```python
from build123d import *

# Parameters (mm, degrees)
BOSS_EXTRUDE1_DEPTH   = 135
RIB3_REACH            = 95.436
SKETCH4_WALL_W        = 207.229173432
SKETCH4_WALL_H        = 3
RIB4_START            = -3
RIB4_DEPTH            = 3
F_6_CLEARANCE_HOLE1_D = 3.7973
SKETCH6_R             = 2.3495
CUT_EXTRUDE1_DEPTH    = 7
SKETCH12_R            = 2.6162
CUT_EXTRUDE2_DEPTH    = 6.35


# Read off the part's stored shape, not the designer's step: Rib4
with BuildPart() as part:
    # Sketch1 → Boss-Extrude1 (new body)
    with BuildSketch(Plane.XY):
        with BuildLine():
            Line((0, 0), (0, 12))
            Line((0, 12), (-8, 12))
            Line((-8, 12), (-8, 6))
            ThreePointArc((-8, 6), (-8.878679656, 3.878679656), (-11, 3))
            Line((-11, 3), (-24, 3))
            Line((-24, 3), (-24, 0))
            Line((-24, 0), (0, 0))
        make_face()
    extrude(amount=BOSS_EXTRUDE1_DEPTH)

    # Sketch4 wall → Rib3 (add, up to next)
    with BuildSketch(Plane(origin=(-16, 7.5, 45.5), x_dir=(-0.871575537125, -0.490261239633, 0), z_dir=(-0.490261239633, 0.871575537125, 0)), mode=Mode.PRIVATE) as rib3_sk1:
        Rectangle(SKETCH4_WALL_W, SKETCH4_WALL_H)
    rib3_tool1 = extrude(rib3_sk1.sketch, amount=-RIB3_REACH, mode=Mode.PRIVATE) - part.part
    rib3 = rib3_tool1.solids().sort_by_distance((-16, 7.5, 45.5))[0]
    add(rib3)

    # Rib4 outline → Rib4 (add)
    with BuildSketch(Plane(origin=(0, 0, 0), x_dir=(-1, 0, 0), z_dir=(0, 0, -1)).offset(RIB4_START)):
        with BuildLine():
            Line((24, 3), (8, 12))
            Line((8, 12), (8, 6))
            ThreePointArc((8, 6), (8.878679656, 3.878679656), (11, 3))
            Line((11, 3), (24, 3))
        make_face()
    rib4 = extrude(amount=RIB4_DEPTH)

    # Mirror1: Rib3, Rib4 across plane
    add(rib3.mirror(Plane(origin=(0, 0, 67.5), x_dir=(1, 0, 0), z_dir=(0, 0, -1))))
    add(rib4.mirror(Plane(origin=(0, 0, 67.5), x_dir=(1, 0, 0), z_dir=(0, 0, -1))))

    # #6 Clearance Hole1 (through all)
    with Locations(Plane(origin=(0, 0, 0), x_dir=(-1, 0, 0), z_dir=(0, -1, 0))):
        with Locations((17.5, -22.5), (17.5, -112.5), (17.5, -67.5)):
            Hole(F_6_CLEARANCE_HOLE1_D / 2)

    # Sketch6 → Cut-Extrude1 (cut)
    with BuildSketch(Plane(origin=(0, 0, 0), x_dir=(0, 0, -1), z_dir=(1, 0, 0))):
        with Locations((-112.5, 6)):
            Circle(SKETCH6_R)
        with Locations((-67.5, 6)):
            Circle(SKETCH6_R)
        with Locations((-22.5, 6)):
            Circle(SKETCH6_R)
    extrude(amount=-CUT_EXTRUDE1_DEPTH, mode=Mode.SUBTRACT)

    # Sketch12 → Cut-Extrude2 (cut)
    with BuildSketch(Plane(origin=(0, 0, 0), x_dir=(0, 0, -1), z_dir=(1, 0, 0))):
        with Locations((-112.5, 6)):
            Circle(SKETCH12_R)
        with Locations((-67.5, 6)):
            Circle(SKETCH12_R)
        with Locations((-22.5, 6)):
            Circle(SKETCH12_R)
    extrude(amount=-CUT_EXTRUDE2_DEPTH, mode=Mode.SUBTRACT)


solid = part.part
```
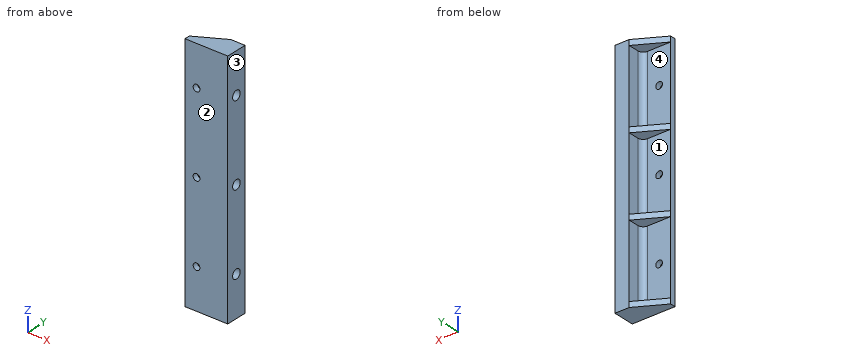
Source: CAD feature listing. Evaluate the final solid. Frame: model axes, mm. Face numbers are marked on the shaded views. A direction names the side the tool comes from. Round coordinates to 2 decimals unless told otherwise and drop trailing zeros. Loops run counter-clockwise (first coordinate to the right, second up) from the corner with the lowest first, then second, coordinate; pieces in that order, holes last.
(1) Section query B-B (z = 112.5). Output: boundary loops of the cut face in (x, y), and give its area (3 significant figures).
From the geometry:
outline: (-24, 0) - (-19.4, 0) - (-19.4, 3) - (-24, 3) - close; (-15.6, 0) - (0, 0) - (0, 3.38) - (-6.35, 3.38) - (-6.35, 3.65) - (-7, 3.65) - (-7, 8.35) - (-6.35, 8.35) - (-6.35, 8.62) - (0, 8.62) - (0, 12) - (-8, 12) - (-8, 6) arc R3 cw to (-11, 3) - (-15.6, 3) - close
area: 98.3 mm2
(2) Contact query for flat-ended pins moving along their axis: pin 1 Ø1.6 at (y, z) = (5, 68.5) entering from +X; pin 2 Ø10.5 at (x, z) = (-20, 109.5) entering from +Y; pin 3 Ø4 at (y, z) = (9.5, 91) entering from -X. Output: stop coordinate, or through.
From the geometry:
pin 1: stops at x = -7
pin 2: stops at y = 3
pin 3: stops at x = -16
(3) Access query for the marked faces 3 and 4. Directions: +Z, -Z, +X, -X, +Y, -Y. A direction counts if a zero-diameter tool reaches every point of the face in a straight line with its end or side. Return the directions, or none.
From the geometry:
face 3: +Z, -Z, +X, +Y, -Y
face 4: -X, +Y
(4) Pull-direction query (Z, two-part tool) for the marked faces 1 and 2; classes: +Z half, -Z half, draft (parallel to the pull), parting line (faces both ways), or undercut.
From the geometry:
face 1: undercut
face 2: draft
(5) Material intervals for probe 1 along Z at (x, y) = (-9, 7.5); probe 2 along Y at (x, z) = (-6.75, 112.5); probe 3 along Z at (x, y) = (-17.5, 1.8), sorted ascending.
From the geometry:
probe 1: z = 0 to 3, 44 to 47, 88 to 91, 132 to 135
probe 2: y = 0 to 3.65, 8.35 to 12
probe 3: z = 0 to 20.6, 24.4 to 65.6, 69.4 to 110.6, 114.4 to 135
(6) Section query A-A (x = -17.5). Output: boundary loops of the cut face in (y, z), and give its area (3 significant figures).
From the geometry:
outline: (0, 0) - (6.66, 0) - (6.66, 3) - (3, 3) - (3, 20.6) - (0, 20.6) - close; (0, 24.4) - (3, 24.4) - (3, 44) - (6.66, 44) - (6.66, 47) - (3, 47) - (3, 65.6) - (0, 65.6) - close; (0, 69.4) - (3, 69.4) - (3, 88) - (6.66, 88) - (6.66, 91) - (3, 91) - (3, 110.6) - (0, 110.6) - close; (0, 114.4) - (3, 114.4) - (3, 132) - (6.66, 132) - (6.66, 135) - (0, 135) - close
area: 415 mm2
(7) Section query C-C (z = 16). Output: boundary loops of the cut face in (x, y).
From the geometry:
outline: (-24, 0) - (0, 0) - (0, 12) - (-8, 12) - (-8, 6) arc R3 cw to (-11, 3) - (-24, 3) - close
(8) Section query D-D (x = -9.5). Output: boundary loops of the cut face in (y, z).
From the geometry:
outline: (0, 0) - (11.16, 0) - (11.16, 3) - (3.4, 3) - (3.4, 44) - (11.16, 44) - (11.16, 47) - (3.4, 47) - (3.4, 88) - (11.16, 88) - (11.16, 91) - (3.4, 91) - (3.4, 132) - (11.16, 132) - (11.16, 135) - (0, 135) - close
